```python
from build123d import *

# Parameters (mm, degrees)
ESQUISSE1_W                  = 50
ESQUISSE1_H                  = 30
BOSS_EXTRU_1_DEPTH           = 10
BOSS_EXTRU_2_DEPTH           = 15
BOSS_EXTRU_2_DEPTH_BACK      = 15
ESQUISSE2_R                  = 2.5
ENL_V_MAT_EXTRU_1_DEPTH      = 10
ENL_V_MAT_EXTRU_1_DEPTH_BACK = 10
ESQUISSE3_R                  = 10.88408721
ESQUISSE3_R_2                = 2.5


with BuildPart() as part:
    # Esquisse1 → Boss.-Extru.1 (new body)
    with BuildSketch(Plane(origin=(0, 0, 0), x_dir=(1, 0, 0), z_dir=(0, 1, 0))):
        Rectangle(ESQUISSE1_W, ESQUISSE1_H)
    extrude(amount=BOSS_EXTRU_1_DEPTH)

    # Esquisse2 → Boss.-Extru.2 (add, two sides: drawn at the far end of the back side and taken through both)
    with BuildSketch(Plane(origin=(0, 0, 0), x_dir=(0, 0, -1), z_dir=(1, 0, 0)).offset(-BOSS_EXTRU_2_DEPTH_BACK)):
        with BuildLine():
            Line((-10, 20), (-10, 10))
            Line((-10, 10), (10, 10))
            Line((10, 10), (10, 20))
            ThreePointArc((10, 20), (0, 30), (-10, 20))
        make_face()
        with Locations((0, 20)):
            Circle(ESQUISSE2_R, mode=Mode.SUBTRACT)
    extrude(amount=BOSS_EXTRU_2_DEPTH + BOSS_EXTRU_2_DEPTH_BACK)

    # Esquisse3 → Enlèv. mat.-Extru.1 (cut, two sides: drawn at the far end of the back side and taken through both)
    with BuildSketch(Plane(origin=(0, 0, 0), x_dir=(0, 0, -1), z_dir=(1, 0, 0)).offset(-ENL_V_MAT_EXTRU_1_DEPTH_BACK)):
        with Locations((0, 20)):
            Circle(ESQUISSE3_R)
        with Locations((0, 20)):
            Circle(ESQUISSE3_R_2, mode=Mode.SUBTRACT)
    extrude(amount=ENL_V_MAT_EXTRU_1_DEPTH + ENL_V_MAT_EXTRU_1_DEPTH_BACK, mode=Mode.SUBTRACT)


solid = part.part
```
Geometry check sheet. Reference: the model listing, model coordinates, mm. A direction names the side the tool comes from. Coordinates: 2 decimals unless noted, no trailing zeros. Order: outer loops, then holes, each group sorted by start corner. A loop starts at its lowest first (then second) coordinate and runs counter-clockwise, first axis right, second up. Notation, with made-up numbers: M -12,86.25 L 25,86.25 A20 ccw 25,111.25 Z; hole C -8.5,51.5 d8. An arc over 180 degrees is marked long. Answer as a JSON object with one key per item and string values.
Q1. Tool access check on faces 5 (the flat face through (-15, 18, -2)), 6 (the flat face through (15, 18, -2)), 7 (the cylindrical face through (-0.14, 9.117, 0.178)), 8 (the flat face through (0, 14, 10)), 9 (the cylindrical face through (12, 30, 0)). Record the directions out of +Z, -Z, +X, -X, +Y, -Y that give a thin tool (end or side, any length) a straight path to the whole face; none if there is none.
Results are:
{"face 5": "+Z, -Z, -X, +Y", "face 6": "+Z, -Z, +X, +Y", "face 7": "+Y", "face 8": "+Z, +X, -X, +Y", "face 9": "+X, -X, +Y"}
Q2. Cross-section at B-B on y = 16.5. Record the cut outline in (x, z).
Results are:
{"outline": "M -15,-10 L -10,-10 L -10,10 L -15,10 Z; M 10,-10 L 15,-10 L 15,10 L 10,10 Z"}
Q3. Cross-section at C-C on x = -8. Record the cut outline in (y, z).
Results are:
{"outline": "M 0,-15 L 10,-15 L 10,-10 L 15.7,-10 A10.88 cw 15.7,10 L 10,10 L 10,15 L 0,15 Z"}
Q4. Release check for a two-part mould opening along Z. For faces 1 (the flat face through (0, 0, 0)), 2 (the cylindrical face through (-13, 30, 0)), 3 (the flat face through (0, 14, -10)), 4 (the flat face through (-10, 17, 0)) record: released by +Z, released by -Z, zero draft, split by the parting line, or undercut.
Results are:
{"face 1": "zero draft", "face 2": "split by the parting line", "face 3": "released by -Z", "face 4": "undercut"}
Q5. Cross-section at D-D on y = 27. Record the cut outline in (x, z).
Results are:
{"outline": "M -15,-7.14 L -10,-7.14 L -10,7.14 L -15,7.14 Z; M 10,-7.14 L 15,-7.14 L 15,7.14 L 10,7.14 Z"}
Q6. Cross-section at A-A on z = 0. Record the cut outline in (x, y).
Results are:
{"outline": "M -25,0 L 25,0 L 25,10 L 15,10 L 15,17.5 L 10,17.5 L 10,9.12 L -10,9.12 L -10,17.5 L -15,17.5 L -15,10 L -25,10 Z; M -15,22.5 L -10,22.5 L -10,30 L -15,30 Z; M 10,22.5 L 15,22.5 L 15,30 L 10,30 Z"}
Q7. Scan lines: line 1 (Y direction, x = 11.45, z = 0); line 2 (X direction, y = 27.75, z = 5.25); line 3 (Y direction, x = -20, z = 11.75). Record each from-to range of solid material in increasing order.
Results are:
{"line 1": "y = 0 to 17.5, 22.5 to 30", "line 2": "x = -15 to -10, 10 to 15", "line 3": "y = 0 to 10"}
Q8. Depth check by flat-ended pin: pin 1 Ø4 at (y, z) = (16.5, -10) entering from -X; pin 2 Ø12 at (x, y) = (13.5, 13.5) entering from +Z; pin 3 Ø16 at (y, z) = (21, 3) entering from +X; pin 4 Ø4 at (y, z) = (20, 0) entering from +X. Enter the tip coordinate at first touch or a pass-through.
Results are:
{"pin 1": "stops at x = -15", "pin 2": "stops at z = 15", "pin 3": "stops at x = 15", "pin 4": "passes through"}
